Check sheet for the modelled part. Datum: model origin and axes. Units: mm. Coordinates: 2 decimals unless noted, no trailing zeros. Loops run counter-clockwise (first coordinate to the right, second up) from the corner with the lowest first, then second, coordinate; pieces in that order, holes last. Notation, with made-up numbers: M -30.5,32 L -6.5,32 A21 cw -6.5,71 Z; hole C -23.5,-1 d3. An arc over 180 degrees is marked long. Answer in a Markdown table with one row per item. Add a question column.
```python
from build123d import *

# Parameters (mm, degrees)
SKETCH1_W                      = 40
SKETCH1_H                      = 39
BOSS_EXTRUDE1_DEPTH            = 1
SKETCH2_W                      = 20
SKETCH2_H                      = 39
BOSS_EXTRUDE2_DEPTH            = 1
FILLET1_R                      = 2
F_1_6_1_6_DIAMETER_HOLE1_D     = 1.6
F_1_6_1_6_DIAMETER_HOLE1_DEPTH = 19.77
F_1_6_1_6_DIAMETER_HOLE1_TIP   = 0.480688495
SKETCH11_R                     = 4.2
CUT_EXTRUDE1_DEPTH             = 7.4
FILLET2_R                      = 1
SKETCH12_R                     = 0.5
CUT_EXTRUDE2_DEPTH             = 10
SKETCH14_R                     = 0.5
CUT_EXTRUDE3_DEPTH             = 10


with BuildPart() as part:
    # Sketch1 → Boss-Extrude1 (new body)
    with BuildSketch(Plane(origin=(0, 0, 0), x_dir=(1, 0, 0), z_dir=(0, 1, 0))):
        Rectangle(SKETCH1_W, SKETCH1_H)
    extrude(amount=BOSS_EXTRUDE1_DEPTH)

    # Sketch2 → Boss-Extrude2 (add)
    with BuildSketch(Plane(origin=(0, 0, 0), x_dir=(1, 0, 0), z_dir=(0, 1, 0))):
        with Locations((-30, 0)):
            Rectangle(SKETCH2_W, SKETCH2_H)
    extrude(amount=BOSS_EXTRUDE2_DEPTH)

    # Fillet1
    fillet1_edges = [part.edges().sort_by_distance(p)[0] for p in [
        (-40, 0.5, -19.5),
        (-40, 0.5, 19.5),
        (20, 0.5, -19.5),
        (20, 0.5, 19.5),
    ]]
    fillet(fillet1_edges, radius=FILLET1_R)

    # Ø1.6 (1.6) Diameter Hole1
    with Locations(Plane(origin=(0, 1, 0), x_dir=(1, 0, 0), z_dir=(0, 1, 0))):
        with Locations((10, 14.58), (10, 4.42), (10, -4.42), (10, -14.58), (-9, -14.58), (-9, -4.42), (-9, 4.42), (-9, 14.58)):
            Hole(F_1_6_1_6_DIAMETER_HOLE1_D / 2, depth=F_1_6_1_6_DIAMETER_HOLE1_DEPTH)
            with Locations((0, 0, -(F_1_6_1_6_DIAMETER_HOLE1_DEPTH + F_1_6_1_6_DIAMETER_HOLE1_TIP / 2))):  # 118° drill point
                Cone(0, F_1_6_1_6_DIAMETER_HOLE1_D / 2, F_1_6_1_6_DIAMETER_HOLE1_TIP, mode=Mode.SUBTRACT)

    # Sketch11 → Cut-Extrude1 (cut)
    with BuildSketch(Plane(origin=(0, 0, 0), x_dir=(1, 0, 0), z_dir=(0, 1, 0))):
        with Locations((-10, -21.5)):
            Circle(SKETCH11_R)
        with Locations((-10, 21.5)):
            Circle(SKETCH11_R)
    extrude(amount=CUT_EXTRUDE1_DEPTH, mode=Mode.SUBTRACT)

    # Fillet2
    fillet2_edges = [part.edges().sort_by_distance(p)[0] for p in [
        (-6.306762937, 0.5, 19.5),
        (-13.693237063, 0.5, 19.5),
        (-13.693237063, 0.5, -19.5),
        (-6.306762937, 0.5, -19.5),
    ]]
    fillet(fillet2_edges, radius=FILLET2_R)

    # Sketch12 → Cut-Extrude2 (cut)
    with BuildSketch(Plane(origin=(0, 0, 0), x_dir=(1, 0, 0), z_dir=(0, 1, 0))):
        with Locations(Location((-32, 10, 0), (0, 0, 270))):
            Circle(SKETCH12_R)
    extrude(amount=CUT_EXTRUDE2_DEPTH, mode=Mode.SUBTRACT)

    # Sketch14 → Cut-Extrude3 (cut)
    with BuildSketch(Plane(origin=(0, 0, 0), x_dir=(1, 0, 0), z_dir=(0, 1, 0))):
        with Locations(Location((-10, 0, 0), (0, 0, 270))):
            Circle(SKETCH14_R)
    extrude(amount=CUT_EXTRUDE3_DEPTH, mode=Mode.SUBTRACT)


solid = part.part
```
Q1. Thickness scan on L1, parallel to X at y = 0.4, z = 14.58; L2, parallel to X at y = 0.4, z = 0; L3, parallel to X at y = 0.5, z = 4. Record the ranges inside material, lowest first.
Q2. Mould release check, pull along X, two halves, no side actions. Record for faces 1 (the face through (-39.43, 0.51, 18.9)), 2 (the face through (10.59, 0.49, 3.88)), 3 (the face through (19.43, 0.51, 18.9)): released by +X, released by -X, zero draft, split by the parting line, or undercut.
Q3. Cross-section at B-B (y = 0.65). Count the separate pieces of the cut face and the enclosed holes in it, plus the area to 3 significant figures.
Q4. Cross-section at A-A (z = -14.58). Record the cut outline in (x, y), plus the area to 3 significant figures.
Q5. Go/stop test with a flat-tipped pin: pin 1 (1.3 mm diameter, centred on x = -9, z = 14.58, fed in from -Y). Record where the tip stops, or that it passes through.
Answer key:
| question | item | result |
|---|---|---|
| 1 | L1 | -40 to -9.8, -8.2 to 9.2, 10.8 to 20 |
| 1 | L2 | -40 to -10.5, -9.5 to 20 |
| 1 | L3 | -40 to -9.68, -8.32 to 9.32, 10.68 to 20 |
| 2 | face 1 | released by -X |
| 2 | face 2 | undercut |
| 2 | face 3 | released by +X |
| 3 | separate pieces | 1 |
| 3 | enclosed holes | 10 |
| 3 | area | 2,300 mm^2 |
| 4 | outline | M -40,0 L -9.8,0 L -9.8,1 L -40,1 Z; M -8.2,0 L 9.2,0 L 9.2,1 L -8.2,1 Z; M 10.8,0 L 20,0 L 20,1 L 10.8,1 Z |
| 4 | area | 56.8 mm^2 |
| 5 | pin 1 | through |
